Autodesk Inventor part; units mm, degrees
ref_plane "YZ Plane" through (0, 0, 0) normal (1, 0, 0) x (0, 1, 0)
ref_plane "XZ Plane" through (0, 0, 0) normal (0, 1, 0) x (-1, 0, 0)
ref_plane "XY Plane" through (0, 0, 0) normal (0, 0, 1) x (1, 0, 0)
sketch "Sketch1" plane through (0, 0, 0) normal (0, 1, 0) x (-1, 0, 0)
  line L0 (-27.6479, 82.55) -> (27.6479, 82.55)
  line L1 (27.6479, 82.55) -> (27.6479, -82.55)
  line L2 (27.6479, -82.55) -> (-27.6479, -82.55)
  line L3 (-27.6479, -82.55) -> (-27.6479, 82.55)
  line L4 (-27.6479, 82.55) -> (27.6479, -82.55) construction
  line L5 (27.6479, 82.55) -> (-27.6479, -82.55) construction
  point P0 (0, 0)
  dimension "BreadboardWidth" = 55.2958
  dimension "BreadboardLength" = 165.1
extrude "Breadboard" add sketch "Sketch1" along normal mid plane 9.398
sketch "Sketch2" plane through (0, 4.699, 0) normal (0, 1, 0) x (1, 0, 0)
  line L0 (12.7, 27.6225) -> (-12.7, 27.6225)
  line L1 (-12.7, 27.6225) -> (-12.7, 80.9625)
  line L2 (-12.7, 80.9625) -> (12.7, 80.9625)
  line L3 (12.7, 80.9625) -> (12.7, 27.6225)
  line L4 (12.7, 27.6225) -> (-12.7, 80.9625) construction
  line L5 (-12.7, 27.6225) -> (12.7, 80.9625) construction
  line L6 (27.6479, 82.55) -> (-27.6479, 82.55)
  point P0 (0, 0)
  point P1 (0, 54.2925)
  dimension "d4" = 25.4
  dimension "d5" = 53.34
  dimension "d6" = 1.5875
extrude "mBed" add sketch "Sketch2" along normal blind 4.2672
sketch "Sketch3" plane through (0, 4.699, 0) normal (0, 1, 0) x (1, 0, 0)
  line L0 (9.525, 1.27) -> (-9.525, 1.27)
  line L1 (-9.525, 1.27) -> (-9.525, 26.035)
  line L2 (-9.525, 26.035) -> (9.525, 26.035)
  line L3 (9.525, 26.035) -> (9.525, 1.27)
  line L4 (9.525, 1.27) -> (-9.525, 26.035) construction
  line L5 (-9.525, 1.27) -> (9.525, 26.035) construction
  line L6 (-12.7, 27.6225) -> (12.7, 27.6225)
  point P0 (0, 0)
  point P1 (0, 13.6525)
  dimension "d9" = 19.05
  dimension "d10" = 24.765
  dimension "d11" = 1.5875
extrude "Bluetooth Chip" add sketch "Sketch3" along normal blind 3.175
properties part number "Breadboard"
Geometry: final body of the model. Coordinates: model frame, mm. A direction names the side the tool comes from. Give positions to 0.01 mm unless a question says otherwise; leave off trailing zeros. Order: outer loops, then holes, each group sorted by start corner. A loop starts at its lowest first (then second) coordinate and runs counter-clockwise, first axis right, second up. Notation, with made-up numbers: (-34, 58) -> (-19, 58) arc R25 cw to (-19, 70) -> close; hole circle Ø5 at (65, 89). An arc over 180 degrees is marked (long way). Write each question's results on one line, items separated by ' | '. Start each with the question number.
1) Section A-A (z = -71). Return loops of the section in (x, y), then the cut area to 3 significant figures.
2) Section C-C (z = -18). Return loops of the section in (x, y) (3 decimals), then the cut area to 3 significant figures.
3) Section D-D (x = 18). Return loops of the section in (y, z).
4) Line query: line 1 (Z direction, x = -5.5, y = 5.25) (1 decimal); line 2 (Y direction, x = -3, z = 56); line 3 (X direction, y = 4.75, z = -48). Output: solid intervals per line, ascending. Write a range as from..to.
5) Draft query along Z for faces 1 (the flat face through (27.648, 0, -1)), 2 (the flat face through (0, 7, -27.622)), 3 (the flat face through (0, 0, -82.55)), 4 (the flat face through (0, 6, -26.035)). Return one class per face: pulls with the +Z half, pulls with the -Z half, needs draft (parallel to the pull), parting line crosses it, or undercut.
6) First-contact query: pin 1 (1 mm diameter, centred on y = 6, z = 57, fed in from -X) (1 decimal); pin 2 (2.5 mm diameter, centred on y = 6, z = -11, fed in from +X) (3 decimals); pin 3 (10 mm diameter, centred on x = 16.5, z = -10, fed in from +Y); pin 4 (2 mm diameter, centred on y = 7, z = -41.5, fed in from -X). Flat tips, straight axial feed; report the tip coordinate or a pass-through.
7) Set-up query: faces 5 (the flat face through (-9.525, 6, -13)), 6 (the flat face through (0, 7, -80.962)), 7 (the flat face through (-12.7, 7, -54)), 8 (the flat face through (12.7, 7, -55)), 9 (the flat face through (0, 6, -1.27)). Return all of +Z, -Z, +X, -X, +Y, -Y with unobstructed straight access to the full face (end or side cutting, diameter ignored); none if empty.
Calculated:
1) outline: (-27.65, -4.7) -> (27.65, -4.7) -> (27.65, 4.7) -> (12.7, 4.7) -> (12.7, 8.97) -> (-12.7, 8.97) -> (-12.7, 4.7) -> (-27.65, 4.7) -> close | area: 628 mm2
2) outline: (-27.648, -4.699) -> (27.648, -4.699) -> (27.648, 4.699) -> (9.525, 4.699) -> (9.525, 7.874) -> (-9.525, 7.874) -> (-9.525, 4.699) -> (-27.648, 4.699) -> close | area: 580 mm2
3) outline: (-4.7, -82.55) -> (4.7, -82.55) -> (4.7, 82.55) -> (-4.7, 82.55) -> close
4) line 1: -81..-27.6, -26..-1.3 | line 2: -4.7..4.7 | line 3: -12.7..12.7
5) face 1: needs draft | face 2: undercut | face 3: pulls with the -Z half | face 4: undercut
6) pin 1: through | pin 2: x = 9.525 | pin 3: y = 4.7 | pin 4: x = -12.7
7) face 5: +Z, -X, +Y | face 6: -Z, +X, -X, +Y | face 7: +Z, -Z, -X, +Y | face 8: +Z, -Z, +X, +Y | face 9: +Z, +X, -X, +Y
